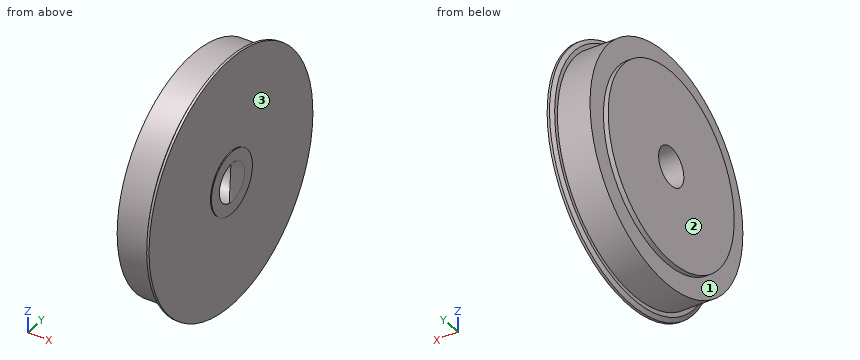
from build123d import *
from build123d.topology import SkipClean

# Parameters (mm, degrees)
PER_AGE1_D         = 8
ESQUISSE13_R       = 6.5
ESQUISSE13_R_2     = 4
BOSS_EXTRU_1_DEPTH = 0.2


with BuildPart() as part:
    # Esquisse1 → Base-Révolution (revolve)
    with BuildSketch(Plane.XY, mode=Mode.PRIVATE) as base_r_volution_sk:
        Polygon((0, 0), (8.8, 0), (8.8, 26), (8.3, 26), (7.8, 25.133974596), (7.8, 24.26), (1, 24.26), (1, 20), (0, 20), align=None)
    revolve(base_r_volution_sk.sketch.rotate(Axis((-7.956160198, 0, 0), (1, 0, 0)), 90), axis=Axis((-7.956160198, 0, 0), (1, 0, 0)))

    # Perçage1 (through all)
    with Locations(Plane(origin=(8.8, 0, 0), x_dir=(0, 0, -1), z_dir=(1, 0, 0))):
        with Locations((0, 0)):
            Hole(PER_AGE1_D / 2)

    # Esquisse13 → Boss.-Extru.1 (add)
    with SkipClean():  # the faces are left unmerged after this step: merging them gives an invalid solid
        with BuildSketch(Plane(origin=(8.8, 0, 0), x_dir=(0, 0, -1), z_dir=(1, 0, 0))):
            Circle(ESQUISSE13_R)
            Circle(ESQUISSE13_R_2, mode=Mode.SUBTRACT)
        extrude(amount=BOSS_EXTRU_1_DEPTH)


solid = part.part
Design review of the part built by this model. Coordinates are the model's own, in mm. Face numbers are marked on the shaded views. A direction names the side the tool comes from. Coordinates: 2 decimals unless noted, no trailing zeros. Order: outer loops, then holes, each group sorted by start corner. A loop starts at its lowest first (then second) coordinate and runs counter-clockwise, first axis right, second up. Notation, with made-up numbers: (-25, 57) - (-20, 57) arc R7 cw to (-20, 69) - close; hole circle Ø5 at (89.5, -22.5). An arc over 180 degrees is marked (long way). Put each result on its own line as item: value.
1) Take a section at B-B, the plane x = 2.5. Give the boundary of the cut face in (y, z).
Response values:
outline: circle Ø48.52 at (0, 0); hole circle Ø8 at (0, 0)
2) Tool access review of the marked faces 1, 2 and 3: name each direction out of +Z, -Z, +X, -X, +Y, -Y from which nothing blocks a thin tool from reaching the whole face with its end or side.
Response values:
face 1: -X
face 2: +Z, -Z, -X, +Y, -Y
face 3: +X
3) Wall thickness on L1, parallel to Y at x = 5.75, z = 0; L2, parallel to X at y = 16, z = 9.5; L3, parallel to X at y = 11.5, z = 20.5: over which ranges is each line inside the solid? List them lowest first. Write a range as from..to.
Response values:
L1: y = -24.26..-4, 4..24.26
L2: x = 0..8.8
L3: x = 1..8.8
4) Insertion check: P1, Ø6, axis at y = -11, z = -18, coming from the +X side; P2, Ø1, axis at x = 5.5, z = -5, coming from the -Y side; P3, Ø1.5, axis at x = 5, y = -19.5, coming from the +Z side. Each pin has a flat end and moves straight along its axis. Give the tip position at first contact, or say it passes through.
Response values:
P1: stops at x = 8.8
P2: stops at y = -23.84
P3: stops at z = 15.39
